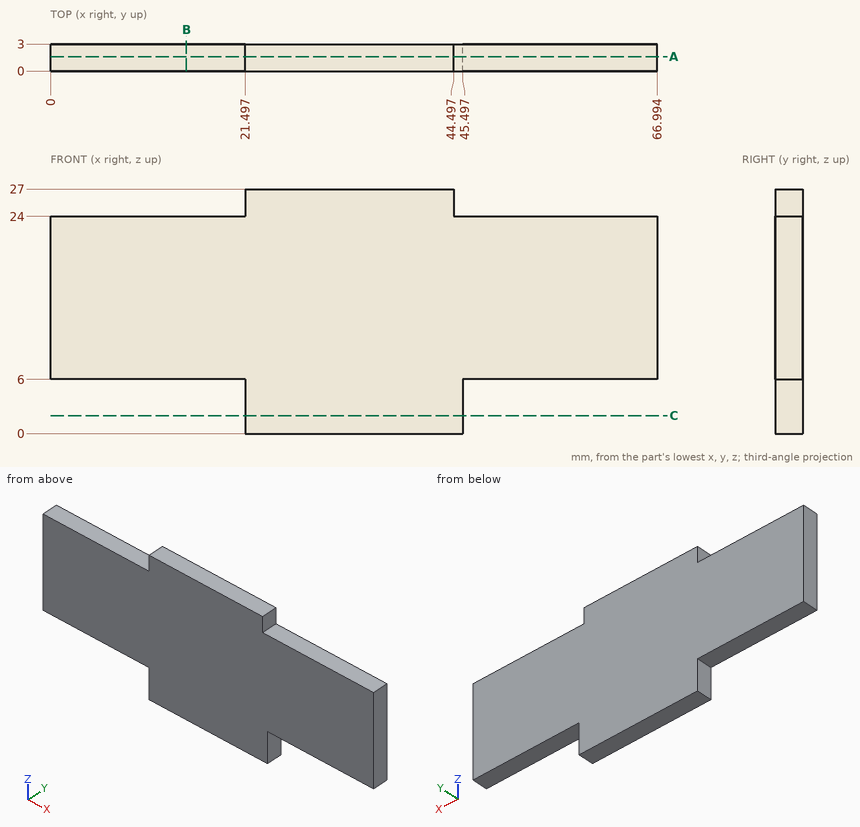
Study the drawing (mm; zero at the part's minimum x, y, z) and answer. Round coordinates to 2 decimals unless told otherwise and drop trailing zeros. Write each loop counter-clockwise with the first axis right and the second up, starting at its lowest first coordinate (ties: lowest second). Pieces come first, ordered by that corner, then holes. Notation, with made-up numbers: (34, -39) - (71, -39) arc R31 cw to (71, -11) - close; hole circle Ø6 at (38.5, -14). An arc over 180 degrees is marked (long way). Use a Markdown table: item, result. Add a question column.
1. The part is cut by section A-A (y = 1.6). Write down the section's boundary in (x, z) (1 decimal).
2. The part is cut by section B-B (x = 15). Write down the section's boundary in (y, z).
3. The part is cut by section C-C (z = 2). Write down the section's boundary in (x, y).
4. Flat-ended cylindrical pins translate along their axes: P1, Ø10, axis at x = 15, z = 19, coming from the -Y side; P2, Ø1.5, axis at y = 1, z = 25.5, coming from the +X side; P3, Ø0.9, axis at x = 8, y = 1, coming from the -Z side; P4, Ø0.9, axis at y = 2, z = 1.5, coming from the +X side. Find the tip coordinate at first contact, or state that the pin passes through.
5. Consider line 1 (X direction, y = 0.6, z = 25.25); line 2 (Z direction, x = 64, y = 0.8); line 3 (X direction, y = 0.7, z = 2.75). Determine where each line is inside the solid, lowest interval first.
Reported:
| question | item | result |
|---|---|---|
| 1 | outline | (0, 6) - (21.5, 6) - (21.5, 0) - (45.5, 0) - (45.5, 6) - (67, 6) - (67, 24) - (44.5, 24) - (44.5, 27) - (21.5, 27) - (21.5, 24) - (0, 24) - close |
| 2 | outline | (0, 6) - (3, 6) - (3, 24) - (0, 24) - close |
| 3 | outline | (21.5, 0) - (45.5, 0) - (45.5, 3) - (21.5, 3) - close |
| 4 | P1 | y = 0 |
| 4 | P2 | x = 44.5 |
| 4 | P3 | z = 6 |
| 4 | P4 | x = 45.5 |
| 5 | line 1 | 21.5 to 44.5 |
| 5 | line 2 | 6 to 24 |
| 5 | line 3 | 21.5 to 45.5 |
